Read the model definition and answer for the solid it produces. Units are mm, in the model's axes. A direction names the side the tool comes from. Coordinates: 2 decimals unless noted, no trailing zeros. Loops run counter-clockwise (first coordinate to the right, second up) from the corner with the lowest first, then second, coordinate; pieces in that order, holes last. Notation, with made-up numbers: (46, 11) - (93, 11) arc R21 ccw to (93, 31) - close; hole circle Ø10 at (56.25, -9). An arc over 180 degrees is marked (long way). Use one line per item in the form item = value.
from build123d import *

# Parameters (mm, degrees)
F0_W      = 150.0394791365
F0_H      = 68.2500004768
F1_DEPTH  = 25
F2_R      = 14.6010069538
F2_R_2    = 14.601
F3_DEPTH  = 86
F4_W      = 73.0581060052
F4_H      = 34.6081331372
F5_DEPTH  = 30
F7_DEPTH  = 50
F9_DEPTH  = 29
F11_DEPTH = 29
F12_R     = 8.621691767
F13_DEPTH = 110.5


# Not quite as in the source:
# - a feature names something its author has since deleted; it is built from what else it names


with BuildPart() as f1:
    # F0 (on Top) → F1 (new body)
    with BuildSketch(Plane.XY):
        Rectangle(F0_W, F0_H)
        with BuildLine():
            Line((-75.0197395682, -34.1250002384), (-75.0197395682, 34.1250002384))
            ThreePointArc((-75.0197395682, 34.1250002384), (-109.1447398067, 0), (-75.0197395682, -34.1250002384))
        make_face()
        with BuildLine():
            ThreePointArc((75.0197395682, -34.1250002384), (109.1447398067, 0), (75.0197395682, 34.1250002384))
            Line((75.0197395682, 34.1250002384), (75.0197395682, -34.1250002384))
        make_face()
    extrude(amount=F1_DEPTH)

    # F2 (on Top) → F3 (cut)
    with BuildSketch(Plane.XY):
        with Locations((-74.1907954216, 0)):
            Circle(F2_R)
        with Locations((76.9539475441, 0)):
            Circle(F2_R_2)
    extrude(amount=F3_DEPTH, mode=Mode.SUBTRACT)

    # F4 (on face) → F5 (join)
    with BuildSketch(Plane.XY.offset(25)):
        Rectangle(F4_W, F4_H)
    extrude(amount=F5_DEPTH)

    # F6 (on face) → F7 (cut)
    with BuildSketch(Plane(origin=(0, 17.3040665686, 0), x_dir=(-1, 0, 0), z_dir=(0, 1, 0))):
        with BuildLine():
            ThreePointArc((-7.6186316787, 35.1906841607), (0, 27.572052482), (7.6186316787, 35.1906841607))
            Line((7.6186316787, 35.1906841607), (-7.6186316787, 35.1906841607))
        make_face()
        with BuildLine():
            Line((-7.6186316787, 35.1906841607), (7.6186316787, 35.1906841607))
            ThreePointArc((7.6186316787, 35.1906841607), (0, 42.8093158393), (-7.6186316787, 35.1906841607))
        make_face()
        with BuildLine():
            ThreePointArc((-7.6186316787, 35.1906841607), (0, 42.8093158393), (7.6186316787, 35.1906841607))
            Line((7.6186316787, 35.1906841607), (7.6186316787, 55))
            Line((7.6186316787, 55), (-7.6186316787, 55))
            Line((-7.6186316787, 55), (-7.6186316787, 35.1906841607))
        make_face()
    extrude(amount=-F7_DEPTH, mode=Mode.SUBTRACT)

    # F8 (on face) → F9 (join)
    with BuildSketch(Plane.YZ.offset(36.5290530026)):
        with BuildLine():
            Line((-17.3040665686, 55), (17.3040665686, 55))
            ThreePointArc((17.3040665686, 55), (0, 72.3040665686), (-17.3040665686, 55))
        make_face()
    extrude(amount=-F9_DEPTH)

    # F10 (on face) → F11 (join)
    with BuildSketch(Plane(origin=(-36.5290530026, 0, 0), x_dir=(0, -1, 0), z_dir=(-1, 0, 0))):
        with BuildLine():
            Line((-17.3040665686, 55), (17.3040665686, 55))
            ThreePointArc((17.3040665686, 55), (0, 72.3040665686), (-17.3040665686, 55))
        make_face()
    extrude(amount=-F11_DEPTH)

    # F12 (on face) → F13 (cut)
    with BuildSketch(Plane(origin=(-36.5290530026, 0, 0), x_dir=(0, -1, 0), z_dir=(-1, 0, 0))):
        with Locations((0, 55)):
            Circle(F12_R)
    extrude(amount=-F13_DEPTH, mode=Mode.SUBTRACT)


solid = f1.part
Item 1: The part is cut by section D-D on z = 14. Give the vertices of the cut face in (x, y) (3 decimals).
Results below:
outline = (-75.02, -34.125) - (75.02, -34.125) arc R34.125 ccw to (75.02, 34.125) - (-75.02, 34.125) arc R34.125 ccw to start; hole circle Ø29.202 at (-74.191, 0); hole circle Ø29.202 at (76.954, 0)
Item 2: The part is cut by section C-C on x = 0. Give the vertices of the cut face in (y, z) (3 decimals), plus the area to 3 significant figures.
Results below:
outline = (-34.125, 0) - (34.125, 0) - (34.125, 25) - (17.304, 25) - (17.304, 27.572) - (-17.304, 27.572) - (-17.304, 25) - (-34.125, 25) - close
area = 1,800 mm²
Item 3: Find the intervals of material crossed by L1, parallel to X at y = 0, z = 12.5; L2, parallel to X at y = 3, z = 9; L3, parallel to X at y = -7, z = 42, in increasing order.
Results below:
L1 = -109.14 to -88.79, -59.59 to 62.35, 91.55 to 109.14
L2 = -109.01 to -88.48, -59.9 to 62.66, 91.24 to 109.01
L3 = -36.53 to -7.62, 7.62 to 36.53
Item 4: Which of the six approach directions +Z, -Z, +X, -X, +Y, -Y give full straight-line access (tool end or side, diameter ignored) to faces 4 (the flat face through (-9, 17.304, 40)), 5 (the flat face through (-36.529, 0, 44)), 6 (the flat face through (-9, -17.304, 40)), 7 (the flat face through (7.529, 0, 64))?
Results below:
face_4 = +Z, +X, -X, +Y
face_5 = +Z, -X, +Y, -Y
face_6 = +Z, +X, -X, -Y
face_7 = +Z, +Y, -Y
Item 5: The part is cut by section A-A on y = 0. Give the vertices of the cut face in (x, z), plus the area to 3 significant figures.
Results below:
outline = (-109.14, 0) - (-88.79, 0) - (-88.79, 25) - (-109.14, 25) - close; (-59.59, 0) - (62.35, 0) - (62.35, 25) - (36.53, 25) - (36.53, 46.38) - (7.62, 46.38) - (7.62, 35.19) arc R7.62 cw to (-7.62, 35.19) - (-7.62, 46.38) - (-36.53, 46.38) - (-36.53, 25) - (-59.59, 25) - close; (-36.53, 63.62) - (-7.53, 63.62) - (-7.53, 72.3) - (-36.53, 72.3) - close; (7.53, 63.62) - (36.53, 63.62) - (36.53, 72.3) - (7.53, 72.3) - close; (91.55, 0) - (109.14, 0) - (109.14, 25) - (91.55, 25) - close
area = 5,800 mm²
Item 6: For a pull along X with two mould halves and no side action, classify faces 1 (the flat face through (7.619, 0, 43)), 2 (the cylindrical face through (-22.232, -4.635, 62.27)), 3 (the cylindrical face through (109.136, -0.75, 12.325)) as +X half, -X half, draft (parallel to the pull), parting line (faces both ways), or undercut.
Results below:
face_1 = undercut
face_2 = draft
face_3 = +X half
Item 7: The part is cut by section B-B on x = -23.5. Give the vertices of the cut face in (y, z) (3 decimals), plus the area to 3 significant figures.
Results below:
outline = (-34.125, 0) - (34.125, 0) - (34.125, 25) - (17.304, 25) - (17.304, 55) arc R17.304 ccw to (-17.304, 55) - (-17.304, 25) - (-34.125, 25) - close; hole circle Ø17.243 at (0, 55)
area = 2,980 mm²
Item 8: Each of these flat-tipped pins is pushed along its axis until it touches: P1, Ø6, axis at y = 18.5, z = 54.5, coming from the +X side; P2, Ø9, axis at x = -10.5, z = 35, coming from the +Y side; P3, Ø1, axis at x = 9, z = 51.5, coming from the -Y side. Where does it stop, or does it pass through?
Results below:
P1 = 36.53
P2 = 17.3
P3 = -17.3
